Geometry: see drawing. Coordinates: mm, zero at the bounding-box minimum. A direction names the side the tool comes from. Round coordinates to 2 decimals unless told otherwise and drop trailing zeros. Loops run counter-clockwise (first coordinate to the right, second up) from the corner with the lowest first, then second, coordinate; pieces in that order, holes last. Notation, with made-up numbers: (44.5, 85) - (50.5, 85) arc R11 ccw to (50.5, 102) - close; hole circle Ø8 at (81, -8.5). An arc over 180 degrees is marked (long way). Answer in a Markdown table with one row per item. Add a question column.
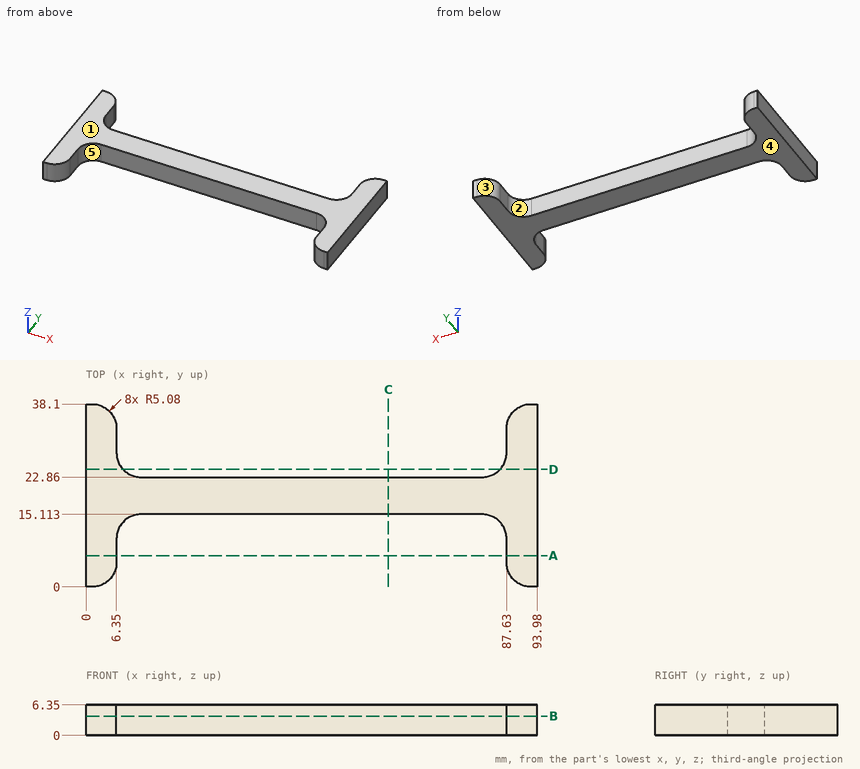
1) Contact query for flat-ended pins moving along their axis: pin 1 Ø10 at (x, y) = (65, 28.5) entering from -Z; pin 2 Ø2.5 at (y, z) = (31, 2) entering from -X; pin 3 Ø1 at (x, z) = (40, 1.5) entering from +Y. Output: stop coordinate, or through.
2) Section A-A, the plane y = 6.5. Return the cut outline in (x, z), and give its area (3 significant figures).
3) Reachability of the marked faces 3, 4 and 5 from +Z, -Z, +X, -X, +Y, -Y: full face, straight path, thin tool, end or side. Return the list, or none.
4) Section B-B, the plane z = 4. Return the cut outline in (x, y), and give its area (3 significant figures).
5) Section C-C, the plane x = 63. Return the cut outline in (y, z).
6) Section D-D, the plane y = 24.5. Return the cut outline in (x, z), and give its area (3 significant figures).
7) Pull-direction query (X, two-part tool) for the marked faces 1 and 2; classes: pulls with the +X half, pulls with the -X half, needs draft (parallel to the pull), parting line crosses it, or undercut.
8) Material intervals for line 1 along X through (y, z) = (7, 3.5); line 2 along Y through (x, z) = (72, 5.25), sorted ascending. Write a range as from..to.
Evaluation:
| question | item | result |
|---|---|---|
| 1 | pin 1 | passes through |
| 1 | pin 2 | stops at x = 0 |
| 1 | pin 3 | stops at y = 22.86 |
| 2 | outline | (0, 0) - (6.35, 0) - (6.35, 6.35) - (0, 6.35) - close; (87.63, 0) - (93.98, 0) - (93.98, 6.35) - (87.63, 6.35) - close |
| 2 | area | 80.6 mm² |
| 3 | face 3 | +Z, -Z, +Y |
| 3 | face 4 | -Z, +X, -X, +Y, -Y |
| 3 | face 5 | +Z, -Z, -Y |
| 4 | outline | (0, 0) - (1.27, 0) arc R5.08 ccw to (6.35, 5.08) - (6.35, 10.03) arc R5.08 cw to (11.43, 15.11) - (82.55, 15.11) arc R5.08 cw to (87.63, 10.03) - (87.63, 5.08) arc R5.08 ccw to (92.71, 0) - (93.98, 0) - (93.98, 38.1) - (92.71, 38.1) arc R5.08 ccw to (87.63, 33.02) - (87.63, 27.94) arc R5.08 cw to (82.55, 22.86) - (11.43, 22.86) arc R5.08 cw to (6.35, 27.94) - (6.35, 33.02) arc R5.08 ccw to (1.27, 38.1) - (0, 38.1) - close |
| 4 | area | 1,110 mm² |
| 5 | outline | (15.11, 0) - (22.86, 0) - (22.86, 6.35) - (15.11, 6.35) - close |
| 6 | outline | (0, 0) - (7.69, 0) - (7.69, 6.35) - (0, 6.35) - close; (86.29, 0) - (93.98, 0) - (93.98, 6.35) - (86.29, 6.35) - close |
| 6 | area | 97.7 mm² |
| 7 | face 1 | needs draft |
| 7 | face 2 | undercut |
| 8 | line 1 | x = 0..6.35, 87.63..93.98 |
| 8 | line 2 | y = 15.11..22.86 |
